```python
from build123d import *

# Parameters (mm, degrees)
F0_W     = 45.72
F0_H     = 25.4
F1_DEPTH = 2.54
F2_W     = 2.54
F2_H     = 16.891
F3_DEPTH = 14.224
F4_W     = 45.72
F4_H     = 1.27
F5_DEPTH = 14.224
F6_W     = 4.572
F6_H     = 1.27
F7_DEPTH = 12.7


with BuildPart() as f1:
    # F0 (on Top) → F1 (new body)
    with BuildSketch(Plane.XY):
        with Locations((14.433108, -4.829161)):
            Rectangle(F0_W, F0_H)
    extrude(amount=F1_DEPTH)

    # F2 (on face) → F3 (join)
    with BuildSketch(Plane.XY.offset(2.54)):
        with Locations((-2.076892, -9.083661)):
            Rectangle(F2_W, F2_H)
        with Locations((30.943108, -9.083661)):
            Rectangle(F2_W, F2_H)
    extrude(amount=F3_DEPTH)

    # F4 (on face) → F5 (join)
    with BuildSketch(Plane.XY.offset(2.54)):
        with Locations((14.433108, 7.235839)):
            Rectangle(F4_W, F4_H)
    extrude(amount=F5_DEPTH)

    # F6 (on face) → F7 (join)
    with BuildSketch(Plane.XY.offset(2.54)):
        with Locations((-6.140892, 2.917839)):
            Rectangle(F6_W, F6_H)
        with Locations((35.007108, 2.917839)):
            Rectangle(F6_W, F6_H)
    extrude(amount=F7_DEPTH)


solid = f1.part
```
Can you work these out from the model? Positions are in its coordinate system, mm. A direction names the side the tool comes from. Give positions to 0.01 mm unless a question says otherwise; leave off trailing zeros. Loops run counter-clockwise (first coordinate to the right, second up) from the corner with the lowest first, then second, coordinate; pieces in that order, holes last. Notation, with made-up numbers: M 29.25,-24.75 L 88.25,-24.75 A32 ccw 88.25,10.25 Z; hole C -15,45 d3. An arc over 180 degrees is marked long. One line per item, written item: value.
(1) We'd pull the mould along Y, two halves only. Please class faces 4 (the face through (13, -17.529, 2)), 5 (the face through (-2, -0.638, 10)), 6 (the face through (-2, -9, 16.764)): released by +Y, released by -Y, zero draft, split by the parting line, or undercut.
Returned:
face 4: released by -Y
face 5: undercut
face 6: zero draft
(2) Suppose I cut it at A-A on z = 9.5. List the corners of the cut face in (x, y) for me.
Returned:
outline: M -8.43,2.28 L -3.85,2.28 L -3.85,3.55 L -8.43,3.55 Z; M -8.43,6.6 L 37.29,6.6 L 37.29,7.87 L -8.43,7.87 Z; M -3.35,-17.53 L -0.81,-17.53 L -0.81,-0.64 L -3.35,-0.64 Z; M 29.67,-17.53 L 32.21,-17.53 L 32.21,-0.64 L 29.67,-0.64 Z; M 32.72,2.28 L 37.29,2.28 L 37.29,3.55 L 32.72,3.55 Z
(3) I need wall thicknesses on line 1 (X direction, y = -14.25, z = 4.25); line 2 (Y direction, x = -4.5, z = 12); line 3 (X direction, y = 2.5, z = 14). Which ranges of each line are inside material? Lowest first, please.
Returned:
line 1: -3.35 to -0.81, 29.67 to 32.21
line 2: 2.28 to 3.55, 6.6 to 7.87
line 3: -8.43 to -3.85, 32.72 to 37.29
(4) Suppose I cut it at C-C on x = 27.5. List the corners of the cut face in (y, z) for me.
Returned:
outline: M -17.53,0 L 7.87,0 L 7.87,16.76 L 6.6,16.76 L 6.6,2.54 L -17.53,2.54 Z
(5) Will these pins go through, and if not, where does the flat tip stop? pin 1 (1.5 mm diameter, centred on x = -1.5, y = -3.5, fed in from -Z); pin 2 (2 mm diameter, centred on x = 9.5, y = -0.5, fed in from +Z); pin 3 (1.5 mm diameter, centred on y = -7.5, z = 11.5, fed in from -X); pin 4 (7 mm diameter, centred on y = -8.5, z = 9.5, fed in from +X).
Returned:
pin 1: z = 0
pin 2: z = 2.54
pin 3: x = -3.35
pin 4: x = 32.21
(6) Which directions (+Z, -Z, +X, -X, +Y, -Y) give clear straight access to the entire face, cutting with the end or side of a thin tool? Please do faces 1 (the face through (-0.807, -9, 10)), 2 (the face through (14, 6.601, 10)), 3 (the face through (-6, 2.283, 9)).
Returned:
face 1: +Z, -Y
face 2: +Z, +X, -X
face 3: +Z, +X, -X, -Y
(7) Suppose I cut it at B-B on y = -5.25. List the corners of the cut face in (x, z) for me, plus the area to 3 significant figures.
Returned:
outline: M -8.43,0 L 37.29,0 L 37.29,2.54 L 32.21,2.54 L 32.21,16.76 L 29.67,16.76 L 29.67,2.54 L -0.81,2.54 L -0.81,16.76 L -3.35,16.76 L -3.35,2.54 L -8.43,2.54 Z
area: 188 mm^2
(8) Suppose I cut it at D-D on y = 4. List the corners of the cut face in (x, z) for me.
Returned:
outline: M -8.43,0 L 37.29,0 L 37.29,2.54 L -8.43,2.54 Z
